```python
from build123d import *
from build123d.topology import SkipClean

# Parameters (mm, degrees)
SKETCH_1_W          = 150
SKETCH_1_H          = 150
EXTRUDE_1_DEPTH     = 3
SKETCH_2_W          = 150
SKETCH_2_H          = 150
SKETCH_2_W_2        = 144
SKETCH_2_H_2        = 144
EXTRUDE_2_DEPTH     = 107.65
SKETCH_3_R          = 31.25
CUT_EXTRUDE_1_DEPTH = 91
SKETCH_4_R          = 6
CUT_EXTRUDE_2_DEPTH = 201.9189451
SKETCH_8_R          = 35
SKETCH_8_R_2        = 31.25
EXTRUDE_4_DEPTH     = 18
SKETCH_9_R          = 1.65
CUT_EXTRUDE_3_DEPTH = 201.9189451
EXTRUDE_5_OUTLINE_W = 3.75
EXTRUDE_5_OUTLINE_H = 3


# Read off the part's stored shape, not the designer's step: the extrude step
with BuildPart() as part:
    # Sketch 1 → Extrude 1 (new body)
    with BuildSketch(Plane(origin=(0, 0, 0), x_dir=(1, 0, 0), z_dir=(0, 1, 0))):
        Rectangle(SKETCH_1_W, SKETCH_1_H)
    extrude(amount=EXTRUDE_1_DEPTH)

    # Sketch 2 → Extrude 2 (add)
    with BuildSketch(Plane(origin=(0, 3, 0), x_dir=(1, 0, 0), z_dir=(0, 1, 0))):
        Rectangle(SKETCH_2_W, SKETCH_2_H)
        Rectangle(SKETCH_2_W_2, SKETCH_2_H_2, mode=Mode.SUBTRACT)
    extrude(amount=EXTRUDE_2_DEPTH)

    # Sketch 3 → Cut-Extrude 1 (cut)
    with BuildSketch(Plane.XZ):
        with Locations(Location((0, 0, 0), (0, 0, 270))):
            Circle(SKETCH_3_R)
    extrude(amount=-CUT_EXTRUDE_1_DEPTH, mode=Mode.SUBTRACT)

    # Sketch 4 → Cut-Extrude 2 (cut, through all)
    with BuildSketch(Plane.ZY.offset(75)):
        with Locations((-20.1, 110.65)):
            Circle(SKETCH_4_R)
    extrude(amount=-CUT_EXTRUDE_2_DEPTH, mode=Mode.SUBTRACT)

    # Sketch 8 → Extrude 4 (add, symmetric)
    with SkipClean():  # the faces are left unmerged after this step: merging them gives an invalid solid
        with BuildSketch(Plane(origin=(0, 3, 0), x_dir=(1, 0, 0), z_dir=(0, 1, 0))):
            with Locations(Location((0, 0, 0), (0, 0, 270))):
                Circle(SKETCH_8_R)
            with Locations(Location((0, 0, 0), (0, 0, 270))):
                Circle(SKETCH_8_R_2, mode=Mode.SUBTRACT)
        extrude(amount=EXTRUDE_4_DEPTH, both=True)
    add(part.part.scale(1), mode=Mode.REPLACE)  # the faces are merged on a copy

    # Sketch 9 → Cut-Extrude 3 (cut, through all)
    with BuildSketch(Plane.ZY.offset(75)):
        with Locations((-40.1, 90.65)):
            Circle(SKETCH_9_R)
        with Locations((-0.1, 90.65)):
            Circle(SKETCH_9_R)
    extrude(amount=-CUT_EXTRUDE_3_DEPTH, mode=Mode.SUBTRACT)

    # Extrude 5 outline → Extrude 5 (revolve)
    with BuildSketch(Plane.XY):
        with Locations((29.375, -13.5)):
            Rectangle(EXTRUDE_5_OUTLINE_W, EXTRUDE_5_OUTLINE_H)
    revolve(axis=Axis((0, 0, 0), (0, 1, 0)))


solid = part.part
```
Here's how the part is built. I have some questions about the finished solid (model axes, mm). A direction names the side the tool comes from. Coordinates: 2 decimals unless noted, no trailing zeros. Order: outer loops, then holes, each group sorted by start corner. A loop starts at its lowest first (then second) coordinate and runs counter-clockwise, first axis right, second up. Notation, with made-up numbers: M -27,5 L -17,5 A25 ccw -17,21 Z; hole C 40,19 d1. An arc over 180 degrees is marked long. Answer as a JSON object with one key per item and string values. Group by question number.
(1) Suppose I cut it at B-B, the plane y = 36.5. Please give me the cut outline in (x, z), then the cut area to 3 significant figures.
(2) Suppose I cut it at D-D, the plane z = 44. Please give me the cut outline in (x, y).
(3) Which directions (+Z, -Z, +X, -X, +Y, -Y) give clear straight access to the entire face, cutting with the end or side of a thin tool? Please do faces 4 (the face through (-18, 0, 32)), 5 (the face through (0, -12, 28)), 6 (the face through (-73.52, 104.65, -20.23)).
(4) For pin 1 (1.5 mm diameter, centred on x = -9, z = 28.5, fed in from +Y); pin 2 (1.5 mm diameter, centred on x = -56.5, z = -36, fed in from +Y); pin 3 (21 mm diameter, centred on x = -10, z = -9.5, fed in from +Y); pin 4 (4.5 mm diameter, centred on y = 90.65, z = -0.1, fed in from -X), each with a flat end and sliding along its axis, tell me the tip position at first contact or that it passes through.
(5) Suppose I cut it at C-C, the plane x = 54. Please give me the cut outline in (y, z).
(6) I need wall thicknesses on probe 1 along X at (y, z) = (12.25, 0); probe 2 along Z at (x, y) = (69, 35.5); probe 3 along Z at (x, y) = (-74.05, 90.65). Which ranges of each line are inside material? Lowest first, please.
(7) Suppose I cut it at A-A, the plane z = 19. Please give me the cut outline in (x, y), then the cut area to 3 significant figures.
(8) If we mould it in two halves opening along X, with no side actions, what happens to faces 1 (the face through (75, 55, 1)), 2 (the face through (29, 21, -13)), 3 (the face through (-22.6, 110.65, -72.4))? For each: released by +X, released by -X, zero draft, split by the parting line, or undercut.
Values found:
{
 "1": {"outline": "M -75,-75 L 75,-75 L 75,75 L -75,75 Z; hole M -72,-72 L 72,-72 L 72,72 L -72,72 Z", "area": "1,760 mm^2"},
 "2": {"outline": "M -75,0 L 75,0 L 75,110.65 L 72,110.65 L 72,3 L -72,3 L -72,110.65 L -75,110.65 Z"},
 "3": {"face 4": "-Y", "face 5": "+Y", "face 6": "+X, -X, +Y"},
 "4": {"pin 1": "stops at y = -12", "pin 2": "stops at y = 3", "pin 3": "passes through", "pin 4": "stops at x = -75"},
 "5": {"outline": "M 0,-75 L 110.65,-75 L 110.65,-72 L 3,-72 L 3,72 L 110.65,72 L 110.65,75 L 0,75 Z"},
 "6": {"probe 1": "x = -75 to -72, -35 to -31.25, 31.25 to 35, 72 to 75", "probe 2": "z = -75 to -72, 72 to 75", "probe 3": "z = -75 to -41.75, -38.45 to -1.75, 1.55 to 75"},
 "7": {"outline": "M -75,0 L -29.39,0 L -29.39,-15 L -19.88,-15 L -19.88,-12 L -24.81,-12 L -24.81,21 L -29.39,21 L -29.39,3 L -72,3 L -72,110.65 L -75,110.65 Z; M 19.88,-15 L 29.39,-15 L 29.39,0 L 75,0 L 75,110.65 L 72,110.65 L 72,3 L 29.39,3 L 29.39,21 L 24.81,21 L 24.81,-12 L 19.88,-12 Z", "area": "1,280 mm^2"},
 "8": {"face 1": "released by +X", "face 2": "undercut", "face 3": "zero draft"}
}
